from build123d import *

# Parameters (mm, degrees)
SKETCH1_W           = 85
SKETCH1_H           = 77
BOSS_EXTRUDE1_DEPTH = 3
SKETCH3_R           = 17.907
SKETCH3_R_2         = 13.97
BOSS_EXTRUDE3_DEPTH = 4.7625
BOSS_EXTRUDE7_DEPTH = 26
SKETCH6_W           = 77
SKETCH6_H           = 7.5
BOSS_EXTRUDE8_DEPTH = 5


with BuildPart() as part:
    # Sketch1 → Boss-Extrude1 (new body)
    with BuildSketch(Plane(origin=(0, 0, 0), x_dir=(1, 0, 0), z_dir=(0, 1, 0))):
        Rectangle(SKETCH1_W, SKETCH1_H)
    extrude(amount=BOSS_EXTRUDE1_DEPTH)

    # Sketch3 → Boss-Extrude3 (add)
    with BuildSketch(Plane(origin=(0, 3, 0), x_dir=(1, 0, 0), z_dir=(0, 1, 0))):
        with Locations((19.133331774, 19.048949964)):
            Circle(SKETCH3_R)
        with Locations((19.133331774, 19.048949964)):
            Circle(SKETCH3_R_2, mode=Mode.SUBTRACT)
        with Locations((-19.133331774, 19.048949964)):
            Circle(SKETCH3_R)
        with Locations((-19.133331774, 19.048949964)):
            Circle(SKETCH3_R_2, mode=Mode.SUBTRACT)
    extrude(amount=BOSS_EXTRUDE3_DEPTH)

    # Sketch4 → Boss-Extrude7 (add)
    with BuildSketch(Plane(origin=(0, 3, 0), x_dir=(1, 0, 0), z_dir=(0, 1, 0))):
        with BuildLine():
            ThreePointArc((-34.668002675, 27.955949964), (-31.887785522, 31.618140813), (-28.266663548, 34.451641278))
            Line((-28.266663548, 34.451641278), (-28.266663548, 36.955949964))
            Line((-28.266663548, 36.955949964), (-38.266663548, 36.955949964))
            Line((-38.266663548, 36.955949964), (-38.266663548, 27.955949964))
            Line((-38.266663548, 27.955949964), (-34.668002675, 27.955949964))
        make_face()
        with BuildLine():
            ThreePointArc((-28.266663548, 3.64625865), (-31.887785522, 6.479759115), (-34.668002675, 10.141949964))
            Line((-34.668002675, 10.141949964), (-38.266663548, 10.141949964))
            Line((-38.266663548, 10.141949964), (-38.266663548, 1.141949964))
            Line((-38.266663548, 1.141949964), (-28.266663548, 1.141949964))
            Line((-28.266663548, 1.141949964), (-28.266663548, 3.64625865))
        make_face()
        with BuildLine():
            Line((0, 10.141949964), (-3.598660873, 10.141949964))
            ThreePointArc((-3.598660873, 10.141949964), (-6.378878026, 6.479759115), (-10, 3.64625865))
            Line((-10, 3.64625865), (-10, 1.141949964))
            Line((-10, 1.141949964), (0, 1.141949964))
            Line((0, 1.141949964), (0, 10.141949964))
        make_face()
        with BuildLine():
            ThreePointArc((10, 3.64625865), (6.378878026, 6.479759115), (3.598660873, 10.141949964))
            Line((3.598660873, 10.141949964), (0, 10.141949964))
            Line((0, 10.141949964), (0, 1.141949964))
            Line((0, 1.141949964), (10, 1.141949964))
            Line((10, 1.141949964), (10, 3.64625865))
        make_face()
        with BuildLine():
            Line((0, 27.955949964), (0, 36.955949964))
            Line((0, 36.955949964), (-10, 36.955949964))
            Line((-10, 36.955949964), (-10, 34.451641278))
            ThreePointArc((-10, 34.451641278), (-6.378878026, 31.618140813), (-3.598660873, 27.955949964))
            Line((-3.598660873, 27.955949964), (0, 27.955949964))
        make_face()
        with BuildLine():
            Line((10, 36.955949964), (0, 36.955949964))
            Line((0, 36.955949964), (0, 27.955949964))
            Line((0, 27.955949964), (3.598660873, 27.955949964))
            ThreePointArc((3.598660873, 27.955949964), (6.378878026, 31.618140813), (10, 34.451641278))
            Line((10, 34.451641278), (10, 36.955949964))
        make_face()
        with BuildLine():
            Line((28.266663548, 36.955949964), (28.266663548, 34.451641278))
            ThreePointArc((28.266663548, 34.451641278), (31.887785522, 31.618140813), (34.668002675, 27.955949964))
            Line((34.668002675, 27.955949964), (38.266663548, 27.955949964))
            Line((38.266663548, 27.955949964), (38.266663548, 36.955949964))
            Line((38.266663548, 36.955949964), (28.266663548, 36.955949964))
        make_face()
        with BuildLine():
            ThreePointArc((34.668002675, 10.141949964), (31.887785522, 6.479759115), (28.266663548, 3.64625865))
            Line((28.266663548, 3.64625865), (28.266663548, 1.141949964))
            Line((28.266663548, 1.141949964), (38.266663548, 1.141949964))
            Line((38.266663548, 1.141949964), (38.266663548, 10.141949964))
            Line((38.266663548, 10.141949964), (34.668002675, 10.141949964))
        make_face()
    extrude(amount=BOSS_EXTRUDE7_DEPTH)

    # Sketch6 → Boss-Extrude8 (add)
    with BuildSketch(Plane.ZY.offset(42.5)):
        with Locations((0, -0.75)):
            Rectangle(SKETCH6_W, SKETCH6_H)
    boss_extrude8 = extrude(amount=BOSS_EXTRUDE8_DEPTH)

    # Mirror1: Boss-Extrude8 across plane
    add(boss_extrude8.mirror(Plane(origin=(0, 0, 0), x_dir=(0, 0, 1), z_dir=(1, 0, 0))))


solid = part.part
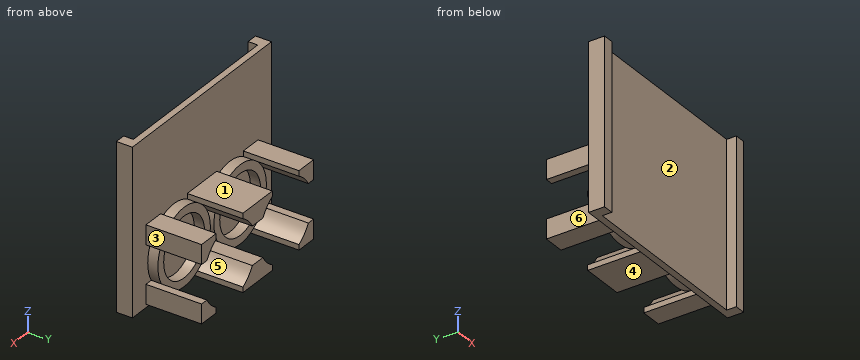
Source: CAD feature listing. Evaluate the final solid. Frame: model axes, mm. Face numbers are marked on the shaded views. A direction names the side the tool comes from. Coordinates: 2 decimals unless noted, no trailing zeros. Loops run counter-clockwise (first coordinate to the right, second up) from the corner with the lowest first, then second, coordinate; pieces in that order, holes last. Notation, with made-up numbers: M 48,32 L 88,32 A11 ccw 88,51 Z; hole C -15,89.25 d7. An arc over 180 degrees is marked long. Answer in a Markdown table with one row per item.
Q1. Section A-A on y = 23. State how many separate pieces and enclosed holes the cut face has, plus the area to 3 significant figures.
Answers below:
| item | result |
|---|---|
| separate pieces | 6 |
| enclosed holes | 0 |
| area | 525 mm^2 |
Q2. Section D-D on x = -12.5. Return the cut outline in (y, z), plus the area to 3 significant figures.
Answers below:
| item | result |
|---|---|
| outline | M 0,-38.5 L 3,-38.5 L 3,-35.68 L 7.76,-35.68 L 7.76,-31.34 L 3,-31.34 L 3,-6.75 L 7.76,-6.75 L 7.76,-2.42 L 3,-2.42 L 3,38.5 L 0,38.5 Z |
| area | 272 mm^2 |
Q3. Set-up query: the marked faces 4, 5 and 6. Return all of +Z, -Z, +X, -X, +Y, -Y with unobstructed straight access to the full face (end or side cutting, diameter ignored); none if empty.
Answers below:
| item | result |
|---|---|
| face 4 | -Z, +X, -X, +Y |
| face 5 | +Y |
| face 6 | +Z, -Z, -X, +Y |
Q4. Section C-C on z = 16. Return the cut outline in (x, y).
Answers below:
| item | result |
|---|---|
| outline | M -47.5,-4.5 L -42.5,-4.5 L -42.5,0 L 42.5,0 L 42.5,-4.5 L 47.5,-4.5 L 47.5,3 L -47.5,3 Z |
Q5. Section B-B on y = -2. Return the cut outline in (x, z).
Answers below:
| item | result |
|---|---|
| outline | M -47.5,-38.5 L -42.5,-38.5 L -42.5,38.5 L -47.5,38.5 Z; M 42.5,-38.5 L 47.5,-38.5 L 47.5,38.5 L 42.5,38.5 Z |
Q6. First-contact query: pin 1 (2.5 mm diameter, centred on y = 13, z = -7, fed in from +X); pin 2 (8 mm diameter, centred on x = -31.5, y = 22, fed in from +Z); pin 3 (8.5 mm diameter, centred on x = 14.5, z = -21, fed in from +Y). Flat tips, straight axial feed; report the tip coordinate or a pass-through.
Answers below:
| item | result |
|---|---|
| pin 1 | stops at x = 38.27 |
| pin 2 | stops at z = -1.14 |
| pin 3 | stops at y = 3 |
Q7. Draft query along X for the marked faces 1, 2 and 3. Return one class per face: pulls with the +X half, pulls with the -X half, needs draft (parallel to the pull), parting line crosses it, or undercut.
Answers below:
| item | result |
|---|---|
| face 1 | needs draft |
| face 2 | undercut |
| face 3 | pulls with the +X half |
Q8. Ray query, probe 1 along X at (y, z) = (-1.5, -30); probe 2 along Z at (x, y) = (19, 7); probe 3 along X at (y, z) = (16.5, -7). Return the intervals inside material, ascending. Write a range as from..to.
Answers below:
| item | result |
|---|---|
| probe 1 | x = -47.5..-42.5, 42.5..47.5 |
| probe 2 | z = -36.96..-33.02, -5.08..-1.14 |
| probe 3 | x = -38.27..-32.38, -5.89..5.89, 32.38..38.27 |
